Could you check a few things on this model? Use its own coordinates, in mm. A direction names the side the tool comes from. Round coordinates to 2 decimals unless told otherwise and drop trailing zeros. Loops run counter-clockwise (first coordinate to the right, second up) from the corner with the lowest first, then second, coordinate; pieces in that order, holes last. Notation, with made-up numbers: (48, -19.75) -> (62, -19.75) arc R24 ccw to (62, 7.25) -> close; hole circle Ø5 at (13.25, -20.5). An arc over 180 degrees is marked (long way). One line per item, written item: value.
```python
from build123d import *

# Parameters (mm, degrees)
CROQUIS1_W              = 101.54
CROQUIS1_H              = 25.72
CROQUIS1_W_2            = 98.34
CROQUIS1_H_2            = 22.52
SALIENTE_EXTRUIR1_DEPTH = 80
CROQUIS2_W              = 98.34
CROQUIS2_H              = 160
CORTAR_EXTRUIR1_DEPTH   = 11.1


with BuildPart() as part:
    # Croquis1 → Saliente-Extruir1 (new, symmetric)
    with BuildSketch(Plane.XY):
        Rectangle(CROQUIS1_W, CROQUIS1_H)
        Rectangle(CROQUIS1_W_2, CROQUIS1_H_2, mode=Mode.SUBTRACT)
    extrude(amount=SALIENTE_EXTRUIR1_DEPTH, both=True)

    # Croquis2 → Cortar-Extruir1 (cut)
    with BuildSketch(Plane(origin=(0, 12.86, 0), x_dir=(1, 0, 0), z_dir=(0, 1, 0))):
        Rectangle(CROQUIS2_W, CROQUIS2_H)
    extrude(amount=-CORTAR_EXTRUIR1_DEPTH, mode=Mode.SUBTRACT)


solid = part.part
```
(1) Please list where these lines run through material, in increasing order: L1, parallel to X at y = 11.5, z = 22; L2, parallel to Y at x = -43, z = -13.5.
Results below:
L1: x = -50.77 to -49.17, 49.17 to 50.77
L2: y = -12.86 to -11.26
(2) Imagine slicing it at A-A on y = -8.25. Write out the boundary of the cut face in (x, z), then the cut area to 3 significant figures.
Results below:
outline: (-50.77, -80) -> (-49.17, -80) -> (-49.17, 80) -> (-50.77, 80) -> close; (49.17, -80) -> (50.77, -80) -> (50.77, 80) -> (49.17, 80) -> close
area: 512 mm²
(3) On a 3-axis mill with a long thin cutter (end or side, diameter ignored), from which of +Z, -Z, +X, -X, +Y, -Y can I reach the whole of each face in a straight line? I mean faces 1 (the face through (50.77, 0, 1)), 2 (the face through (-1, -11.26, 1)). Say none if no direction works.
Results below:
face 1: +Z, -Z, +X, +Y, -Y
face 2: +Z, -Z, +Y
(4) For pin 1 Ø3 at (x, z) = (-31, 40) entering from +Y, with a flat end and sliding along its axis, tell me the tip position at first contact or that it passes through.
Results below:
pin 1: stops at y = -11.26
(5) Imagine slicing it at B-B on z = -53. Write out the boundary of the cut face in (x, y).
Results below:
outline: (-50.77, -12.86) -> (50.77, -12.86) -> (50.77, 12.86) -> (49.17, 12.86) -> (49.17, -11.26) -> (-49.17, -11.26) -> (-49.17, 12.86) -> (-50.77, 12.86) -> close
(6) We'd pull the mould along X, two halves only. Please class faces 3 (the face through (-1, -12.86, 1)), 4 (the face through (-50.77, 0, 1)), 5 (the face through (-49.17, 1, 1)): +X half, -X half, draft (parallel to the pull), parting line (faces both ways), or undercut.
Results below:
face 3: draft
face 4: -X half
face 5: undercut
(7) Imagine slicing it at C-C on x = -36. Write out the boundary of the cut face in (y, z), then the cut area to 3 significant figures.
Results below:
outline: (-12.86, -80) -> (-11.26, -80) -> (-11.26, 80) -> (-12.86, 80) -> close
area: 256 mm²
